from build123d import *

# Parameters (mm, degrees)
F0_W     = 156
F0_H     = 69.000003
F0_R     = 1
F0_W_2   = 37
F0_H_2   = 2
F1_DEPTH = 2
F2_DEPTH = 8
F3_R     = 1
F4_R     = 2


with BuildPart() as f1:
    # F0 (on Top) → F1 (new body)
    with BuildSketch(Plane.XY):
        with Locations((26.202309, 3.732657)):
            Rectangle(F0_W, F0_H)
        Polygon((-49.797689, 36.232657), (102.202308, 36.232657), (102.202308, -28.767343), (34.202309, -28.767343), (-2.797691, -28.767343), (-49.797689, -28.767343), align=None, mode=Mode.SUBTRACT)
        Polygon((102.202308, -28.767343), (102.202308, 36.232657), (-49.797689, 36.232657), (-49.797689, -28.767343), (-2.797691, -28.767343), (-2.797691, -26.767343), (-47.797689, -26.767343), (-47.797689, 34.232657), (100.202308, 34.232657), (100.202308, -26.767343), (34.202309, -26.767343), (34.202309, -28.767343), align=None)
        Polygon((-2.797691, -26.767343), (34.202309, -26.767343), (100.202308, -26.767343), (100.202308, 34.232657), (-47.797689, 34.232657), (-47.797689, -26.767343), align=None)
        with Locations((-40.572589, 10.712606)):
            Circle(F0_R, mode=Mode.SUBTRACT)
        with Locations((-35.572589, 29.712606)):
            Circle(F0_R, mode=Mode.SUBTRACT)
        with Locations((92.977207, 10.712606)):
            Circle(F0_R, mode=Mode.SUBTRACT)
        with Locations((87.977207, 29.712606)):
            Circle(F0_R, mode=Mode.SUBTRACT)
        with Locations((15.702309, -27.767343)):
            Rectangle(F0_W_2, F0_H_2)
    extrude(amount=-F1_DEPTH)

    # F0 (on Top) → F2 (join)
    with BuildSketch(Plane.XY):
        Polygon((102.202308, -28.767343), (102.202308, 36.232657), (-49.797689, 36.232657), (-49.797689, -28.767343), (-2.797691, -28.767343), (-2.797691, -26.767343), (-47.797689, -26.767343), (-47.797689, 34.232657), (100.202308, 34.232657), (100.202308, -26.767343), (34.202309, -26.767343), (34.202309, -28.767343), align=None)
    extrude(amount=F2_DEPTH)

    # F3
    f3_edges = [f1.edges().sort_by_distance(p)[0] for p in [
        (-51.797691, 38.232658, -1),
        (-51.797691, -30.767345, -1),
        (104.202309, -30.767345, -1),
        (104.202309, 38.232658, -1),
        (34.202309, -27.767343, 8),
        (-2.797691, -27.767343, 8),
        (34.202309, -27.767343, 0),
        (-2.797691, -27.767343, 0),
    ]]
    fillet(f3_edges, radius=F3_R)

    # F4
    f4_edges = [f1.edges().sort_by_distance(p)[0] for p in [
        (-49.797689, -28.767343, 4),
        (102.202308, -28.767343, 4),
        (102.202308, 36.232657, 4),
        (-49.797689, 36.232657, 4),
    ]]
    fillet(f4_edges, radius=F4_R)


solid = f1.part
Geometry: final body of the model. Coordinates: model frame, mm. A direction names the side the tool comes from. Give positions to 0.01 mm unless a question says otherwise; leave off trailing zeros. Write each loop counter-clockwise with the first axis right and the second up, starting at its lowest first coordinate (ties: lowest second). Pieces come first, ordered by that corner, then holes. Notation, with made-up numbers: (1, 33) -> (40, 33) arc R23 ccw to (40, 55) -> close; hole circle Ø9 at (77, -17.5). An arc over 180 degrees is marked (long way). Answer as a JSON object with one key per item and string values.
1. Cut plane B-B on y = 25. Output: boundary loops of the cut face in (x, z), and give its area (3 significant figures).
Ans:
{"outline": "(-51.8, -2) -> (104.2, -2) -> (104.2, 0) -> (102.2, 0) -> (102.2, 8) -> (100.2, 8) -> (100.2, 0) -> (-47.8, 0) -> (-47.8, 8) -> (-49.8, 8) -> (-49.8, 0) -> (-51.8, 0) -> close", "area": "344 mm^2"}
2. Mould query, pull axis X, two halves, no side actions, for faces 5 (the flat face through (25, 34.233, 4)), 6 (the flat face through (-49.798, 4, 4)), 7 (the flat face through (66, -28.767, 4)). Classes: pulls with the +X half, pulls with the -X half, needs draft (parallel to the pull), parting line crosses it, or undercut.
Ans:
{"face 5": "undercut", "face 6": "pulls with the -X half", "face 7": "needs draft"}
3. Cut plane A-A on z = 3. Output: boundary loops of the cut face in (x, y), and give its area (3 significant figures).
Ans:
{"outline": "(-49.8, -26.77) arc R2 ccw to (-47.8, -28.77) -> (-2.8, -28.77) -> (-2.8, -26.77) -> (-47.8, -26.77) -> (-47.8, 34.23) -> (100.2, 34.23) -> (100.2, -26.77) -> (34.2, -26.77) -> (34.2, -28.77) -> (100.2, -28.77) arc R2 ccw to (102.2, -26.77) -> (102.2, 34.23) arc R2 ccw to (100.2, 36.23) -> (-47.8, 36.23) arc R2 ccw to (-49.8, 34.23) -> close", "area": "775 mm^2"}
4. Contact query for flat-ended pins moving along their axis: pin 1 (5 mm diameter, centred on y = 11, z = 1.5, fed in from +X); pin 2 (4 mm diameter, centred on x = 70.5, z = 4, fed in from +Y); pin 3 (1.5 mm diameter, centred on y = -9, z = 6.5, fed in from +X); pin 4 (0.6 mm diameter, centred on y = -28, z = 5, fed in from -X). Output: stop coordinate, or through.
Ans:
{"pin 1": "stops at x = 104.2", "pin 2": "stops at y = 36.23", "pin 3": "stops at x = 102.2", "pin 4": "stops at x = -49.57"}
5. Ray query, probe 1 along X at (y, z) = (10.5, -1); probe 2 along X at (y, z) = (14, 1.5); probe 3 along Y at (x, z) = (92, 0.25). Return the intervals inside material, ascending. Write a range as from..to.
Ans:
{"probe 1": "x = -51.8..-41.55, -39.6..92, 93.95..104.2", "probe 2": "x = -49.8..-47.8, 100.2..102.2", "probe 3": "y = -28.77..-26.77, 34.23..36.23"}
6. Cut plane C-C on x = -30. Output: boundary loops of the cut face in (y, z), and give its area (3 significant figures).
Ans:
{"outline": "(-30.77, -2) -> (38.23, -2) -> (38.23, 0) -> (36.23, 0) -> (36.23, 8) -> (34.23, 8) -> (34.23, 0) -> (-26.77, 0) -> (-26.77, 8) -> (-28.77, 8) -> (-28.77, 0) -> (-30.77, 0) -> close", "area": "170 mm^2"}
7. Access query for faces 1 (the flat face through (27, 36.233, 4)), 2 (the flat face through (67, -26.767, 4)), 3 (the flat face through (102.202, 3, 4)), 4 (the flat face through (-25, -28.767, 4)). Directions: +Z, -Z, +X, -X, +Y, -Y. A direction counts if a zero-diameter tool reaches every point of the face in a straight line with its end or side. Return the directions, or none.
Ans:
{"face 1": "+Z, +X, -X, +Y", "face 2": "+Z", "face 3": "+Z, +X, +Y, -Y", "face 4": "+Z, +X, -X, -Y"}
